Design review of the part shown in the three views and the two pictorial views. Dimensions are in mm from the part's minimum x, y and z. A direction names the side the tool comes from. Give positions to 0.01 mm unless a question says otherwise; leave off trailing zeros. Write each loop counter-clockwise with the first axis right and the second up, starting at its lowest first coordinate (ties: lowest second). Pieces come first, ordered by that corner, then holes. Notation, with made-up numbers: M 8,19 L 16,19 A21 cw 16,30 Z; hole C -5.75,71.25 d2. An arc over 180 degrees is marked long. Write item = value, one per line.
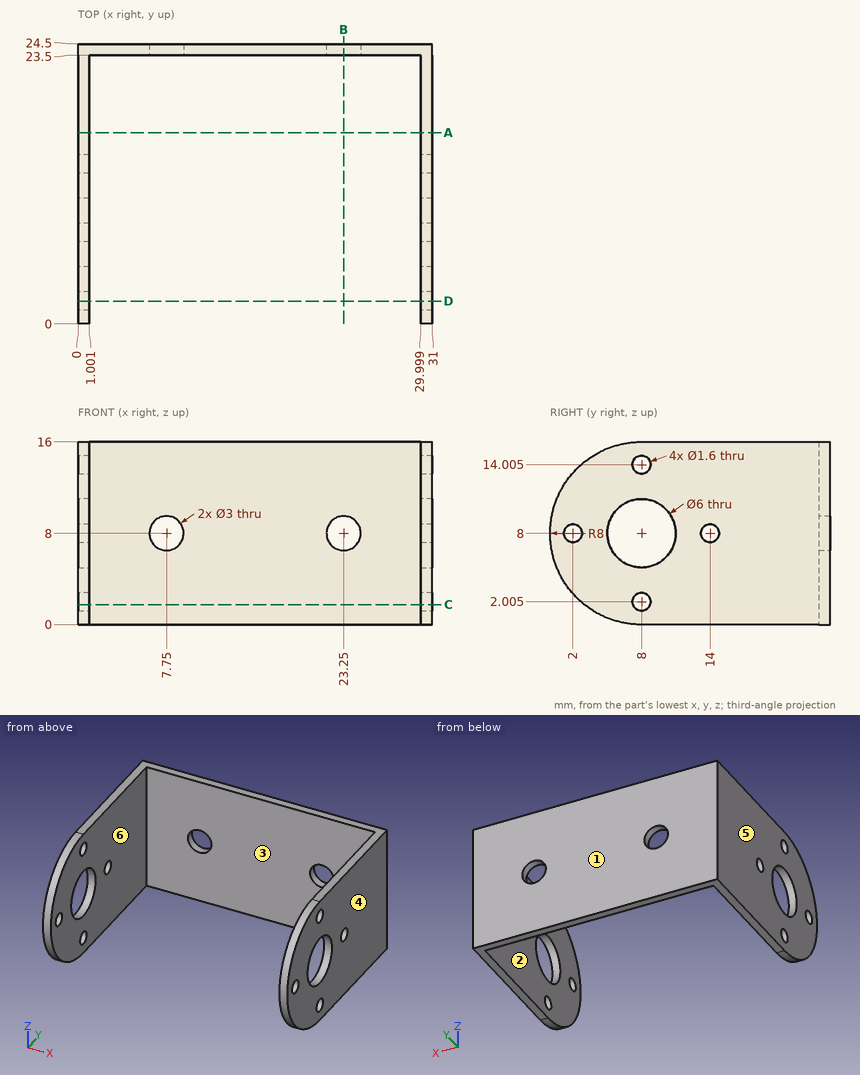
1. For line 1 along Y through (x, z) = (30.65, 8); line 2 along Z through (x, y) = (30.45, 8) (1 decimal); line 3 along X through (y, z) = (4, 6), list the stretches that pass through material, from the lowest coordinate up. Write a range as from..to.
Responses:
line_1 = 0..1.2, 2.8..5, 11..13.2, 14.8..24.5
line_2 = 0..1.2, 2.8..5, 11..13.2, 14.8..16
line_3 = 0..1, 30..31
2. Machinability: for the marked faces 5 and 6, which of the approach directions +Z, -Z, +X, -X, +Y, -Y give a long, thin tool a straight path to every point of the face, cutting with its end or side? Answer none if there is none.
Responses:
face_5 = +Z, -Z, -X, +Y, -Y
face_6 = +Z, -Z, -Y
3. We need section B-B, the plane x = 23.25. Write out the cut boundary in (y, z).
Responses:
outline = M 23.5,0 L 24.5,0 L 24.5,6.5 L 23.5,6.5 Z; M 23.5,9.5 L 24.5,9.5 L 24.5,16 L 23.5,16 Z
4. We need section A-A, the plane y = 16.75. Write out the cut boundary in (x, z).
Responses:
outline = M 0,0 L 1,0 L 1,16 L 0,16 Z; M 30,0 L 31,0 L 31,16 L 30,16 Z
5. We need section C-C, the plane z = 1.75. Write out the cut boundary in (x, y).
Responses:
outline = M 0,3.01 L 1,3.01 L 1,7.24 L 0,7.24 Z; M 0,8.76 L 1,8.76 L 1,23.5 L 30,23.5 L 30,8.76 L 31,8.76 L 31,24.5 L 0,24.5 Z; M 30,3.01 L 31,3.01 L 31,7.24 L 30,7.24 Z
6. Insertion check: P1, Ø1, axis at y = 2, z = 8, coming from the -X side. The pin has a flat end and moves straight along its axis. Give the tip position at first contact, or say it passes through.
Responses:
P1 = through
7. We need section D-D, the plane y = 2. Write out the cut boundary in (x, z), then the cut area to 3 significant figures.
Responses:
outline = M 0,2.71 L 1,2.71 L 1,7.2 L 0,7.2 Z; M 0,8.8 L 1,8.8 L 1,13.29 L 0,13.29 Z; M 30,2.71 L 31,2.71 L 31,7.2 L 30,7.2 Z; M 30,8.8 L 31,8.8 L 31,13.29 L 30,13.29 Z
area = 18.0 mm2
8. The part is to be moulded in two halves that separate along X. For the marked faces 1, 2, 3 and 4, say which applies: +X half, -X half, draft (parallel to the pull), parting line (faces both ways), or undercut.
Responses:
face_1 = draft
face_2 = undercut
face_3 = undercut
face_4 = +X half
